Check sheet for the modelled part. Datum: model origin and axes. Units: mm. A direction names the side the tool comes from. Give positions to 0.01 mm unless a question says otherwise; leave off trailing zeros. Order: outer loops, then holes, each group sorted by start corner. A loop starts at its lowest first (then second) coordinate and runs counter-clockwise, first axis right, second up.
```python
from build123d import *

# Parameters (mm, degrees)
SKETCH1_W                                           = 241.3
SKETCH1_H                                           = 22
BASE_FLANGE_DEPTH                                   = 1
EDGE_FLANGE_MOUNING_STRIP_W                         = 5.4732
EDGE_FLANGE_MOUNING_STRIP_H                         = 1
EDGE_FLANGE_MOUNING_STRIP_CUT_DEPTH                 = 219.8
EDGE_FLANGE_MOUNING_RELIEF_W                        = 5.9732
EDGE_FLANGE_MOUNING_RELIEF_H                        = 0.5
EDGE_FLANGE_MOUNING_RELIEF_CUT_DEPTH                = 1
EDGE_FLANGE_MOUNING_DEPTH                           = 219.8
CUT_EXTRUDE_MOUNTING_DEPTH                          = 1
CSK_FOR_M3_COUNTERSUNK_FLAT_HEAD_SCREW5_D           = 3.2
CSK_FOR_M3_COUNTERSUNK_FLAT_HEAD_SCREW5_CSINK_D     = 6.3
CSK_FOR_M3_COUNTERSUNK_FLAT_HEAD_SCREW5_CSINK_ANGLE = 90
CSK_FOR_M3_COUNTERSUNK_FLAT_HEAD_SCREW6_D           = 3.2
CSK_FOR_M3_COUNTERSUNK_FLAT_HEAD_SCREW6_CSINK_D     = 6.3
CSK_FOR_M3_COUNTERSUNK_FLAT_HEAD_SCREW6_CSINK_ANGLE = 90


# Sheet-metal steps are written as plain solids
with BuildPart() as part:
    # Sketch1 → Base-Flange (new body)
    with BuildSketch(Plane.XY):
        with Locations((-120.65, 11)):
            Rectangle(SKETCH1_W, SKETCH1_H)
    extrude(amount=-BASE_FLANGE_DEPTH)

    # Edge-Flange-Mouning strip (across the edge) → Edge-Flange-Mouning strip cut (cut)
    with BuildSketch(Plane(origin=(-219.8, 22, -1), x_dir=(0, -1, 0), z_dir=(1, 0, 0))):
        with Locations((-1, -0.5)):
            Rectangle(EDGE_FLANGE_MOUNING_STRIP_W, EDGE_FLANGE_MOUNING_STRIP_H)
    extrude(amount=EDGE_FLANGE_MOUNING_STRIP_CUT_DEPTH, mode=Mode.SUBTRACT)

    # Edge-Flange-Mouning relief (on the sheet) → Edge-Flange-Mouning relief cut (cut)
    with BuildSketch(Plane(origin=(-219.8, 20.2634, -1), x_dir=(0, -1, 0), z_dir=(0, 0, -1))):
        with Locations((-2.4866, 0.25)):
            Rectangle(EDGE_FLANGE_MOUNING_RELIEF_W, EDGE_FLANGE_MOUNING_RELIEF_H)
    extrude(amount=-EDGE_FLANGE_MOUNING_RELIEF_CUT_DEPTH, mode=Mode.SUBTRACT)

    # Edge-Flange-Mouning section (across the edge) → Edge-Flange-Mouning (add)
    with BuildSketch(Plane(origin=(-219.8, 22, -1), x_dir=(0, -1, 0), z_dir=(1, 0, 0))):
        with BuildLine():
            Line((0, 0.7366), (0, 9))
            Line((0, 9), (1, 9))
            Line((1, 9), (1, 0.7366))
            ThreePointArc((1, 0.7366), (1.215745145, 0.215745145), (1.7366, 0))
            Line((1.7366, 0), (1.7366, -1))
            ThreePointArc((1.7366, -1), (0.508638364, -0.491361636), (0, 0.7366))
        make_face()
    extrude(amount=EDGE_FLANGE_MOUNING_DEPTH)

    # Sketch13 → Cut-Extrude-Mounting (cut)
    with BuildSketch(Plane.XY):
        with BuildLine():
            Line((-229.5, 12.9), (-235.5, 12.9))
            ThreePointArc((-235.5, 12.9), (-238.5, 15.9), (-235.5, 18.9))
            Line((-235.5, 18.9), (-229.5, 18.9))
            ThreePointArc((-229.5, 18.9), (-226.5, 15.9), (-229.5, 12.9))
        make_face()
    extrude(amount=-CUT_EXTRUDE_MOUNTING_DEPTH, mode=Mode.SUBTRACT)

    # Mirror-Vertical: part across plane


with BuildPart() as part_1:
    add(part.part)
    add(part.part.mirror(Plane(origin=(0, 0, -1), x_dir=(0, 0, 1), z_dir=(1, 0, 0))))

    # Mirror-Horizontal: part across face


with BuildPart() as part_2:
    add(part_1.part)
    add(part_1.part.mirror(Plane(origin=(0, 0, -0.5), x_dir=(0, 0, 1), z_dir=(0, -1, 0))))

    # CSK for M3 Countersunk Flat Head Screw5 (through all)
    with Locations(Plane(origin=(0, 22, 0), x_dir=(1, 0, 0), z_dir=(0, 1, 0))):
        with Locations((-212.4317, 5.8683), (212.4317, 5.8683)):
            CounterSinkHole(CSK_FOR_M3_COUNTERSUNK_FLAT_HEAD_SCREW5_D / 2, CSK_FOR_M3_COUNTERSUNK_FLAT_HEAD_SCREW5_CSINK_D / 2, counter_sink_angle=CSK_FOR_M3_COUNTERSUNK_FLAT_HEAD_SCREW5_CSINK_ANGLE)

    # CSK for M3 Countersunk Flat Head Screw6 (through all)
    with Locations(Plane(origin=(0, -22, 0), x_dir=(-1, 0, 0), z_dir=(0, -1, 0))):
        with Locations((-212.4317, 5.8683), (212.4317, 5.8683)):
            CounterSinkHole(CSK_FOR_M3_COUNTERSUNK_FLAT_HEAD_SCREW6_D / 2, CSK_FOR_M3_COUNTERSUNK_FLAT_HEAD_SCREW6_CSINK_D / 2, counter_sink_angle=CSK_FOR_M3_COUNTERSUNK_FLAT_HEAD_SCREW6_CSINK_ANGLE)


solid = part_2.part
```
Q1. Tool access check on faces 1 (the flat face through (3, 21, -6)), 2 (the flat face through (3, 22, -6)). Record the directions out of +Z, -Z, +X, -X, +Y, -Y that give a thin tool (end or side, any length) a straight path to the whole face; none if there is none.
Q2. Material ranges on line 1 (Y direction, x = 105.5, z = -8.5); line 2 (Z direction, x = 3, y = -20); line 3 (Y direction, x = 77, z = -0.25), recorded low to high.
Q3. Draft check along Y on faces 3 (the flat face through (3, -22, -6)), 4 (the flat face through (3, 0, -1)), 5 (the flat face through (3, 0, 0)). Enter one of: pulls with the +Y half, pulls with the -Y half, needs draft (parallel to the pull), parting line crosses it, or undercut.
Q4. Go/stop test with flat-tipped pins: P1, Ø3, axis at x = -97, y = 5, coming from the +Z side; P2, Ø1.8, axis at y = -21, z = -4, coming from the +X side; P3, Ø1.1, axis at y = -20.5, z = -5.5, coming from the -X side. Record where each tip stops, or that it passes through.
Q5. Sectioned sample at A-A, the plane x = -122. Record the cut outline in (y, z).
Q6. Sectioned sample at B-B, the plane y = -5. Record the cut outline in (x, z), plus the area to 3 significant figures.
Filled in:
1. face 1: -Z, +X, -X
1. face 2: +Z, -Z, +X, -X, +Y
2. line 1: y = -22 to -21, 21 to 22
2. line 2: z = -1 to 0
2. line 3: y = -21.16 to 21.16
3. face 3: pulls with the -Y half
3. face 4: undercut
3. face 5: needs draft
4. P1: stops at z = 0
4. P2: stops at x = 219.8
4. P3: stops at x = -219.8
5. outline: (-22, -10) - (-21, -10) - (-21, -1.74) arc R0.74 cw to (-20.26, -1) - (20.26, -1) arc R0.74 cw to (21, -1.74) - (21, -10) - (22, -10) - (22, -1.74) arc R1.74 ccw to (20.26, 0) - (-20.26, 0) arc R1.74 ccw to (-22, -1.74) - close
6. outline: (-241.3, -1) - (241.3, -1) - (241.3, 0) - (-241.3, 0) - close
6. area: 483 mm2
